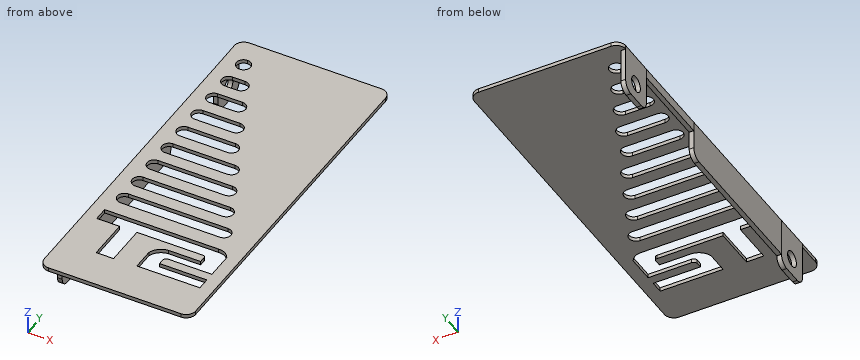
from build123d import *

# Parameters (mm, degrees)
F1_DEPTH = 1.2
F2_DEPTH = 15
F4_D     = 5
F5_R     = 3
F6_DEPTH = 3
F7_DEPTH = 12
F8_R     = 3


# Not quite as in the source:
# - a feature names something its author has since deleted; it is built from what else it names


with BuildPart() as f1:
    # F0 (on Top) → F1 (new body)
    with BuildSketch(Plane.XY):
        Polygon((24, 57.25), (-24, 57.25), (-24.0091441598, 54.25), (-22.5091511277, 54.2454279414), (-22.5091511277, 42.2454279414), (-22.5059426621, 15.2501562063), (-22.5, -34.75), (-22.5, -46.75), (-24, -46.75), (-24, -57.25), (24, -57.25), align=None)
        with BuildLine():
            Line((13.9209458456, -22.2416133583), (-17.6390541544, -22.2416133583))
            ThreePointArc((-17.6390541544, -22.2416133583), (-19.8890541544, -19.9916133583), (-17.6390541544, -17.7416133583))
            Line((-17.6390541544, -17.7416133583), (13.9209458456, -17.7416133583))
            ThreePointArc((13.9209458456, -17.7416133583), (16.1709458456, -19.9916133583), (13.9209458456, -22.2416133583))
        make_face(mode=Mode.SUBTRACT)
        with BuildLine():
            Line((9.9809458456, -13.7416133583), (-17.6390541544, -13.7416133583))
            ThreePointArc((-17.6390541544, -13.7416133583), (-19.8890541544, -11.4916133583), (-17.6390541544, -9.2416133583))
            Line((-17.6390541544, -9.2416133583), (9.9809458456, -9.2416133583))
            ThreePointArc((9.9809458456, -9.2416133583), (12.2309458456, -11.4916133583), (9.9809458456, -13.7416133583))
        make_face(mode=Mode.SUBTRACT)
        with BuildLine():
            Line((6.0409458456, -5.2416133583), (-17.6390541544, -5.2416133583))
            ThreePointArc((-17.6390541544, -5.2416133583), (-19.8890541544, -2.9916133583), (-17.6390541544, -0.7416133583))
            Line((-17.6390541544, -0.7416133583), (6.0409458456, -0.7416133583))
            ThreePointArc((6.0409458456, -0.7416133583), (8.2909458456, -2.9916133583), (6.0409458456, -5.2416133583))
        make_face(mode=Mode.SUBTRACT)
        with BuildLine():
            Line((-19.9999999992, -31.5317022603), (-19.9999999992, -27.0317022603))
            Line((-19.9999999992, -27.0317022603), (16.0951670268, -27.0317022603))
            ThreePointArc((16.0951670268, -27.0317022603), (18.3824934665, -27.555243649), (19.9999999704, -29.25513498))
            Line((19.9999999704, -29.25513498), (19.991580365, -37.75513498))
            Line((19.991580365, -37.75513498), (6.1573753969, -37.7551350426))
            ThreePointArc((6.1573753969, -37.7551350426), (5.4441089744, -38.037790108), (4.9890264818, -38.6554816172))
            Line((4.9890264818, -38.6554816172), (4.9890264818, -40.6197120801))
            Line((4.9890264818, -40.6197120801), (19.9890264818, -40.6197120801))
            Line((19.9890264818, -40.6197120801), (20, -44.6197120801))
            Line((20, -44.6197120801), (0, -44.6197120801))
            Line((0, -44.6197120801), (0, -37.7900532508))
            ThreePointArc((0, -37.7900532508), (1.5958871284, -35.3350022858), (4.3312619815, -34.2900834468))
            Line((4.3312619815, -34.2900834468), (14.5000001306, -34.2900834468))
            Line((14.5000001306, -34.2900834468), (14.5000000048, -32.3122422563))
            ThreePointArc((14.5000000048, -32.3122422563), (14.2713851276, -31.7603171319), (13.7194600008, -31.5317022603))
            Line((13.7194600008, -31.5317022603), (-7.2499999992, -31.5317022603))
            Line((-7.2499999992, -31.5317022603), (-7.2499999992, -44.8960133593))
            Line((-7.2499999992, -44.8960133593), (-12.7499999992, -44.8960133593))
            Line((-12.7499999992, -44.8960133593), (-12.7499999992, -31.5317022603))
            Line((-12.7499999992, -31.5317022603), (-19.9999999992, -31.5317022603))
        make_face(mode=Mode.SUBTRACT)
        with BuildLine():
            Line((2.1009458456, 3.2583866417), (-17.6390541544, 3.2583866417))
            ThreePointArc((-17.6390541544, 3.2583866417), (-19.8890541544, 5.5083866417), (-17.6390541544, 7.7583866417))
            Line((-17.6390541544, 7.7583866417), (2.1009458456, 7.7583866417))
            ThreePointArc((2.1009458456, 7.7583866417), (4.3509458456, 5.5083866417), (2.1009458456, 3.2583866417))
        make_face(mode=Mode.SUBTRACT)
        with BuildLine():
            Line((-2.5590541544, 11.7583866417), (-17.6390541544, 11.7583866417))
            ThreePointArc((-17.6390541544, 11.7583866417), (-19.8890541544, 14.0083866417), (-17.6390541544, 16.2583866417))
            Line((-17.6390541544, 16.2583866417), (-2.5590541544, 16.2583866417))
            ThreePointArc((-2.5590541544, 16.2583866417), (-0.3090541544, 14.0083866417), (-2.5590541544, 11.7583866417))
        make_face(mode=Mode.SUBTRACT)
        with BuildLine():
            Line((-5.7790541544, 20.2583866417), (-17.6390541544, 20.2583866417))
            ThreePointArc((-17.6390541544, 20.2583866417), (-19.8890541544, 22.5083866417), (-17.6390541544, 24.7583866417))
            Line((-17.6390541544, 24.7583866417), (-5.7790541544, 24.7583866417))
            ThreePointArc((-5.7790541544, 24.7583866417), (-3.5290541544, 22.5083866417), (-5.7790541544, 20.2583866417))
        make_face(mode=Mode.SUBTRACT)
        with BuildLine():
            Line((-9.7190541544, 28.7583866417), (-17.6390541544, 28.7583866417))
            ThreePointArc((-17.6390541544, 28.7583866417), (-19.8890541544, 31.0083866417), (-17.6390541544, 33.2583866417))
            Line((-17.6390541544, 33.2583866417), (-9.7190541544, 33.2583866417))
            ThreePointArc((-9.7190541544, 33.2583866417), (-7.4690541544, 31.0083866417), (-9.7190541544, 28.7583866417))
        make_face(mode=Mode.SUBTRACT)
        with BuildLine():
            Line((-13.6590541544, 37.2583866417), (-17.6390541544, 37.2583866417))
            ThreePointArc((-17.6390541544, 37.2583866417), (-19.8890541544, 39.5083866417), (-17.6390541544, 41.7583866417))
            Line((-17.6390541544, 41.7583866417), (-13.6590541544, 41.7583866417))
            ThreePointArc((-13.6590541544, 41.7583866417), (-11.4090541544, 39.5083866417), (-13.6590541544, 37.2583866417))
        make_face(mode=Mode.SUBTRACT)
        with BuildLine():
            Line((-17.5990541544, 45.7583866417), (-17.6390541544, 45.7583866417))
            ThreePointArc((-17.6390541544, 45.7583866417), (-19.8890541544, 48.0083866417), (-17.6390541544, 50.2583866417))
            Line((-17.6390541544, 50.2583866417), (-17.5990541544, 50.2583866417))
            ThreePointArc((-17.5990541544, 50.2583866417), (-15.3490541544, 48.0083866417), (-17.5990541544, 45.7583866417))
        make_face(mode=Mode.SUBTRACT)
    extrude(amount=-F1_DEPTH)

    # F0 (on Top) → F2 (join)
    with BuildSketch(Plane.XY):
        Polygon((-22.5091511277, 54.2454279414), (-24.0091441598, 54.25), (-23.9357289877, 42.2454279414), (-22.5091511277, 42.2454279414), align=None)
        Polygon((-23.997312058, -34.750000301), (-24, -46.75), (-22.5, -46.75), (-22.5, -34.75), align=None)
    extrude(amount=-F2_DEPTH)

    # F4 (through all)
    with Locations(Plane.YZ):
        with Locations((-40.75, -9.5), (48.25, -9.5)):
            Hole(F4_D / 2)

    # F5
    f5_edges = [f1.edges().sort_by_distance(p)[0] for p in [
        (-23.22244, 42.245428, -15),
        (-23.259148, 54.247714, -15),
        (-23.248656, -34.75, -15),
        (-23.25, -46.75, -15),
    ]]
    fillet(f5_edges, radius=F5_R)

    # F0 (on Top) → F6 (join)
    with BuildSketch(Plane.XY):
        Polygon((-22.5091511277, 42.2454279414), (-23.9357289877, 42.2454279414), (-23.9573206897, 15.2499837059), (-22.5059426621, 15.2501562063), align=None)
    extrude(amount=-F6_DEPTH)

    # F0 (on Top) → F7 (join)
    with BuildSketch(Plane.XY):
        Polygon((-22.5059426621, 15.2501562063), (-23.9573206897, 15.2499837059), (-23.997312058, -34.750000301), (-22.5, -34.75), align=None)
    extrude(amount=-F7_DEPTH)

    # F8
    f8_edges = [f1.edges().sort_by_distance(p)[0] for p in [
        (-23.231632, 15.25007, -12),
        (24, 57.25, -0.6),
        (-24, 57.25, -0.6),
        (-24, -57.25, -0.6),
        (24, -57.25, -0.6),
    ]]
    fillet(f8_edges, radius=F8_R)


solid = f1.part
Here's how the part is built. I have some questions about the finished solid (model axes, mm). Round coordinates to 2 decimals unless told otherwise and drop trailing zeros. Order: outer loops, then holes, each group sorted by start corner. A loop starts at its lowest first (then second) coordinate and runs counter-clockwise, first axis right, second up. Notation, with made-up numbers: M 20,10 L 71,10 A6 cw 71,15 Z; hole C 50,7.5 d6. An arc over 180 degrees is marked long. Return JSON: item names as keys, results as strings. Group by question number.
1. I'm going to push flat-ended pins straight in: pin 1 Ø1.3 at (y, z) = (-40, -0.5) entering from -X; pin 2 Ø8 at (y, z) = (48.25, -9.5) entering from +X; pin 3 Ø5 at (x, y) = (-13, -6.5) entering from -Z. Where does each tip first touch, or does it pass through?
2. If we section it at B-B on y = -16.5: List the corners of the cut face in (x, z) for me, then the cut area to 3 significant figures.
3. If we section it at A-A on y = 48.25: List the corners of the cut face in (x, z) for me, then the cut area to 3 significant figures.
4. Please list where these lines run through material, in increasing order: probe 1 along Z at (x, y) = (-22.75, -40.75); probe 2 along Z at (x, y) = (16, 8.5); probe 3 along Y at (x, z) = (-23.65, -9.5).
Reply:
{
 "1": {"pin 1": "x = -24", "pin 2": "x = -22.51", "pin 3": "z = -1.2"},
 "2": {"outline": "M -23.98,-12 L -22.5,-12 L -22.5,-1.2 L 24,-1.2 L 24,0 L -23.98,0 Z", "area": "73.6 mm^2"},
 "3": {"outline": "M -23.97,-15 L -22.51,-15 L -22.51,-12 L -23.97,-12 Z; M -23.97,-7 L -22.51,-7 L -22.51,-1.2 L -19.88,-1.2 L -19.88,0 L -23.97,0 Z; M -15.36,-1.2 L 24,-1.2 L 24,0 L -15.36,0 Z", "area": "65.0 mm^2"},
 "4": {"probe 1": "-15 to -12, -7 to 0", "probe 2": "-1.2 to 0", "probe 3": "-46.75 to -43.25, -38.25 to 15.21, 42.25 to 45.75, 50.75 to 54.25"}
}
